Can you work these out from the model? Positions are in its coordinate system, mm. Face numbers are marked on the shaded views. Give positions to 0.01 mm unless a question says otherwise; leave off trailing zeros. Order: outer loops, then holes, each group sorted by start corner. A loop starts at its lowest first (then second) coordinate and runs counter-clockwise, first axis right, second up. Notation, with made-up numbers: (-36, 56) - (-1, 56) arc R11 ccw to (-1, 61) - close; hole circle Ø10 at (6, -31.5). An arc over 180 degrees is marked (long way). One line per question, with ' | ' between items.
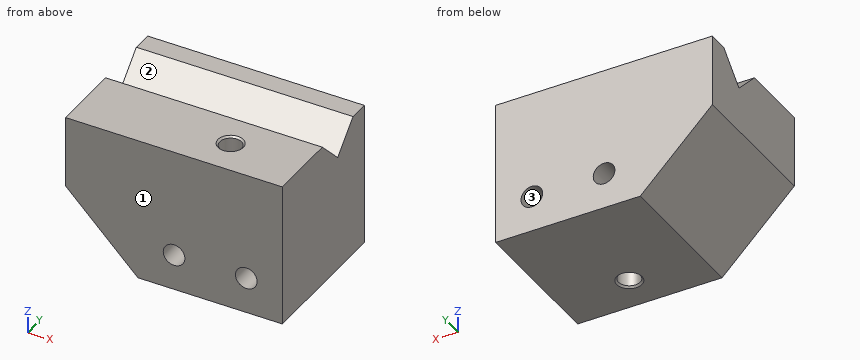
```python
from build123d import *

# Parameters (mm, degrees)
ESQUISSE1_W           = 30
ESQUISSE1_H           = 20
EXTRUSION1_DEPTH      = 20
EXTRUSION2_DEPTH      = 38.416573868
EXTRUSION2_DEPTH_BACK = 38.416573868
ESQUISSE3_R           = 1.5
EXTRUSION3_DEPTH      = 33.015621187
CHANFREIN1_SIZE       = 10


with BuildPart() as part:
    # Esquisse1 → Extrusion1 (new body)
    with BuildSketch(Plane.XY):
        Rectangle(ESQUISSE1_W, ESQUISSE1_H)
    extrude(amount=EXTRUSION1_DEPTH)

    # Esquisse2 → Extrusion2 (cut, two sides: drawn at the far end of the back side and taken through both)
    with BuildSketch(Plane.ZY.offset(15).offset(-EXTRUSION2_DEPTH_BACK)):
        Polygon((64.422439942, 51.672439942), (20, 7.25), (16.25, 3.5), (20, -0.25), (64.422439942, -44.672439942), (190.068074021, -44.672439942), (190.068074021, 51.672439942), align=None)
    extrude(amount=EXTRUSION2_DEPTH + EXTRUSION2_DEPTH_BACK, mode=Mode.SUBTRACT)

    # Esquisse3 → Extrusion3 (cut, through all)
    with BuildSketch(Plane(origin=(0, 10, 0), x_dir=(1, 0, 0), z_dir=(0, 1, 0))):
        with Locations(Location((10, -5, 0), (0, 0, 270))):
            Circle(ESQUISSE3_R)
        with Locations(Location((0, -5, 0), (0, 0, 270))):
            Circle(ESQUISSE3_R)
    extrude(amount=-EXTRUSION3_DEPTH, mode=Mode.SUBTRACT)

    # Chanfrein1
    chanfrein1_edges = [part.edges().sort_by_distance(p)[0] for p in [
        (-15, 0, 0),
    ]]
    chamfer(chanfrein1_edges, length=CHANFREIN1_SIZE)

    # Esquisse4 → Trou taraudé M31 (revolve, cut)
    with BuildSketch(Plane(origin=(5, -5, 20), x_dir=(0, -1, 0), z_dir=(1, 0, 0))):
        Polygon((0, 0), (0, 20), (1.75, 20), (1.5, 19.75), (1.5, 0.25), (1.75, 0), align=None)
    revolve(axis=Axis((5, -5, 26.35), (0, 0, -1)), mode=Mode.SUBTRACT)


solid = part.part
```
(1) Imagine slicing it at D-D (z = 17.75). List the corners of the cut face in (x, y) for me, and give its area (3 significant figures).
Answer below:
outline: (-15, -10) - (15, -10) - (15, 2) - (-15, 2) - close; (-15, 5) - (15, 5) - (15, 10) - (-15, 10) - close; hole circle Ø3 at (5, -5) | area: 503 mm^2
(2) Will these pins go through, and if not, where does the flat tip stop? pin 1 (2.5 mm diameter, centred on x = 10, z = 5, fed in from -Y); pin 2 (3 mm diameter, centred on x = 3, y = 4.5, fed in from +Z); pin 3 (1 mm diameter, centred on y = 6.5, z = 9, fed in from -X).
Answer below:
pin 1: through | pin 2: z = 18.75 | pin 3: x = -14.5
(3) Imagine slicing it at B-B (x = 5). List the corners of the cut face in (y, z) for me.
Answer below:
outline: (-10, 0) - (-6.75, 0) - (-6.5, 0.25) - (-6.5, 19.75) - (-6.75, 20) - (-10, 20) - close; (-3.5, 0.25) - (-3.25, 0) - (10, 0) - (10, 20) - (7.25, 20) - (3.5, 16.25) - (-0.25, 20) - (-3.25, 20) - (-3.5, 19.75) - close
(4) Imagine slicing it at A-A (z = 5). List the corners of the cut face in (x, y) for me, and give its area (3 significant figures).
Answer below:
outline: (-10, -10) - (-1.5, -10) - (-1.5, 10) - (-10, 10) - close; (1.5, -10) - (8.5, -10) - (8.5, 10) - (1.5, 10) - close; (11.5, -10) - (15, -10) - (15, 10) - (11.5, 10) - close; hole circle Ø3 at (5, -5) | area: 373 mm^2
(5) Imagine slicing it at C-C (y = -1.75). List the corners of the cut face in (x, z) for me, and give its area (3 significant figures).
Answer below:
outline: (-15, 10) - (-5, 0) - (15, 0) - (15, 20) - (-15, 20) - close; hole circle Ø3 at (0, 5); hole circle Ø3 at (10, 5) | area: 536 mm^2
(6) If we mould it in two halves opening along Y, with no side actions, what happens to the marked faces 1, 2 and 3? For each: released by +Y, released by -Y, zero draft, split by the parting line, or undercut.
Answer below:
face 1: released by -Y | face 2: undercut | face 3: zero draft
(7) If I drill on line 1 (X direction, y = -2, z = 5); line 2 (Y direction, x = 5, z = 13.5); line 3 (X direction, y = 4.25, z = 4.75), over which ranges is the centre line in solid material (lowest first)?
Answer below:
line 1: -10 to -1.5, 1.5 to 8.5, 11.5 to 15 | line 2: -10 to -6.5, -3.5 to 10 | line 3: -9.75 to -1.48, 1.48 to 8.52, 11.48 to 15
